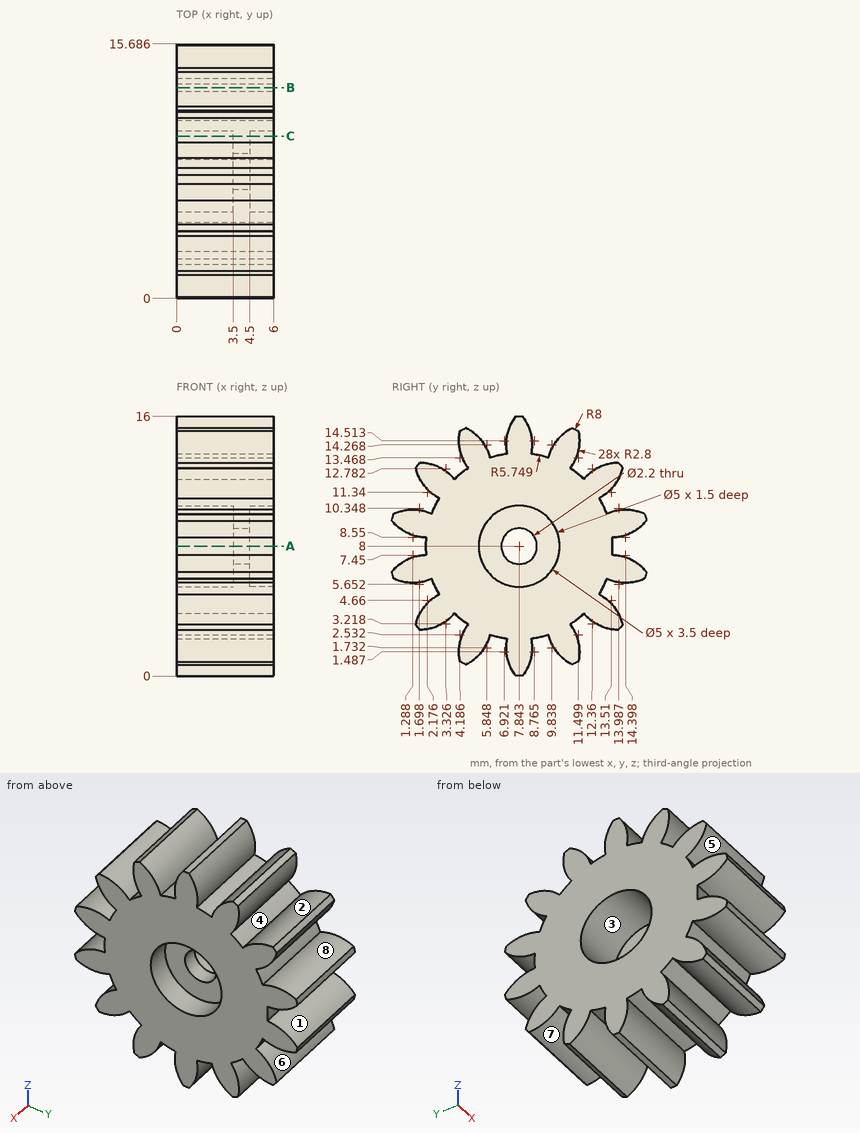
Drawing for the job (mm, zero at the part's lowest x, y, z). A direction names the side the tool comes from. Give positions to 0.01 mm unless a question says otherwise; leave off trailing zeros. Order: outer loops, then holes, each group sorted by start corner. A loop starts at its lowest first (then second) coordinate and runs counter-clockwise, first axis right, second up. Notation, with made-up numbers: M 32,32 L 52,32 A36 cw 52,67 Z; hole C 67.5,15.5 d9. An arc over 180 degrees is marked long. Use a Markdown table: item, result. Add a question column.
(1) Saw through at A-A, the plane z = 8. Give the cut face in (x, y).
(2) Saw through at C-C, the plane y = 10. Give the cut face in (x, z).
(3) Drop flat-ended pins along their axis: P1, Ø3, axis at x = 4.5, y = 5, coming from the +Z side (1 decimal); P2, Ø3, axis at y = 7.84, z = 8, coming from the -X side; P3, Ø4, axis at y = 9, z = 8.5, coming from the -X side; P4, Ø1, axis at x = 3.5, y = 5.5, coming from the +Z side (1 decimal). Give the stop position or say it passes through.
(4) Saw through at B-B, the plane y = 13. Give the cut face in (x, z).
(5) 3-axis set-ups, long thin cutter, end or side, ignore diameter. For the marked faces 1, 2, 3 and 4: which of +Z, -Z, +X, -X, +Y, -Y reach the whole face in a straight line?
(6) Probe line 1 along Z through (x, y) = (1.6, 7.75); line 2 along Y through (x, z) = (4.3, 8); line 3 along Z through (x, y) = (3.15, 13.5) (1 decimal). List the from-to ranges inside material, lowest first. Write a range as [from, to].
(7) Mould opens along Y. For the marked faces 5, 6, 7 and 8 say: +Y half, -Y half, draft (parallel to the pull), parting line (faces both ways), or undercut.
Answer key:
| question | item | result |
|---|---|---|
| 1 | outline | M 0,2.09 L 6,2.09 L 6,5.34 L 4.5,5.34 L 4.5,6.74 L 3.5,6.74 L 3.5,5.34 L 0,5.34 Z; M 0,10.34 L 3.5,10.34 L 3.5,8.94 L 4.5,8.94 L 4.5,10.34 L 6,10.34 L 6,13.59 L 0,13.59 Z |
| 2 | outline | M 0,1.71 L 6,1.71 L 6,6.74 L 4.5,6.74 L 4.5,9.26 L 6,9.26 L 6,14.29 L 0,14.29 L 0,9.26 L 3.5,9.26 L 3.5,6.74 L 0,6.74 Z |
| 3 | P1 | z = 15.3 |
| 3 | P2 | x = 3.5 |
| 3 | P3 | x = 0 |
| 3 | P4 | z = 15 |
| 4 | outline | M 0,3.03 L 6,3.03 L 6,4.9 L 0,4.9 Z; M 0,5.46 L 6,5.46 L 6,10.54 L 0,10.54 Z; M 0,11.1 L 6,11.1 L 6,12.97 L 0,12.97 Z |
| 5 | face 1 | +X, -X, +Y |
| 5 | face 2 | +Z, +X, -X |
| 5 | face 3 | -X |
| 5 | face 4 | +X, -X |
| 6 | line 1 | [0, 5.5], [10.5, 16] |
| 6 | line 2 | [2.09, 6.74], [8.94, 13.59] |
| 6 | line 3 | [2.9, 4.5], [5.9, 10.1], [11.5, 13.1] |
| 7 | face 5 | -Y half |
| 7 | face 6 | +Y half |
| 7 | face 7 | undercut |
| 7 | face 8 | undercut |
